```python
from build123d import *

# Parameters (mm, degrees)
EXTRUDE_2_DEPTH     = 70
CUT_EXTRUDE_1_DEPTH = 90
EXTRUDE_3_OUTLINE_R = 45
EXTRUDE_3_DEPTH     = 20
EXTRUDE_START       = -10
EXTRUDE_4_DEPTH     = 10
EXTRUDE_START_2     = -20
EXTRUDE_5_DEPTH     = 20
CUT_EXTRUDE_2_DEPTH = 207.942020866
EXTRUDE_START_3     = 35
SKETCH_13_R         = 50
EXTRUDE_6_DEPTH     = 35
CUT_EXTRUDE_START   = 15
CUT_EXTRUDE_3_DEPTH = 15
SKETCH_15_R         = 6.5
CUT_EXTRUDE_4_DEPTH = 207.942020866
CUT_EXTRUDE_5_REACH = 207.305


# Read off the part's stored shape, not the designer's step: the extrude step
with BuildPart() as part:
    # Sketch 1 → Extrude 2 (new body)
    with BuildSketch(Plane(origin=(0, 0, 0), x_dir=(1, 0, 0), z_dir=(0, 1, 0))):
        with BuildLine():
            Line((8.235294118, 69.513883008), (92.058823529, 59.583328292))
            ThreePointArc((92.058823529, 59.583328292), (145, 0), (92.058823529, -59.583328292))
            Line((92.058823529, -59.583328292), (8.235294118, -69.513883008))
            ThreePointArc((8.235294118, -69.513883008), (-70, 0), (8.235294118, 69.513883008))
        make_face()
    extrude(amount=EXTRUDE_2_DEPTH)

    # Sketch 2 → Cut-Extrude 1 (cut)
    with BuildSketch(Plane(origin=(0, 70, 0), x_dir=(1, 0, 0), z_dir=(0, 1, 0))):
        with BuildLine():
            Line((7.058823529, -59.583328292), (90.882352941, -49.652773577))
            ThreePointArc((90.882352941, -49.652773577), (135, 0), (90.882352941, 49.652773577))
            Line((90.882352941, 49.652773577), (7.058823529, 59.583328292))
            ThreePointArc((7.058823529, 59.583328292), (-60, 0), (7.058823529, -59.583328292))
        make_face()
    extrude(amount=-CUT_EXTRUDE_1_DEPTH, mode=Mode.SUBTRACT)



with BuildPart() as body_2:
    # Extrude 3 outline → Extrude 3 (new body)
    with BuildSketch(Plane.XZ):
        with BuildLine():
            ThreePointArc((90.882352941, -49.652773577), (135, 0), (90.882352941, 49.652773577))
            Line((90.882352941, 49.652773577), (68.128593603, 52.348406339))
            ThreePointArc((68.128593603, 52.348406339), (30, 0), (68.128593603, -52.348406339))
            Line((68.128593603, -52.348406339), (90.882352941, -49.652773577))
        make_face()
        with Locations((85, 0)):
            Circle(EXTRUDE_3_OUTLINE_R, mode=Mode.SUBTRACT)
    extrude(amount=EXTRUDE_3_DEPTH)


with BuildPart() as part_1:
    add(part.part)

    add(body_2.part)  # Extrude 4 merges body 2
    # Sketch 8 → Extrude 4 (add)
    with BuildSketch(Plane.XZ.offset(EXTRUDE_START)):
        with BuildLine():
            Line((90.882352941, -49.652773577), (7.058823529, -59.583328292))
            ThreePointArc((7.058823529, -59.583328292), (-60, 0), (7.058823529, 59.583328292))
            Line((7.058823529, 59.583328292), (90.882352941, 49.652773577))
            ThreePointArc((90.882352941, 49.652773577), (135, 0), (90.882352941, -49.652773577))
        make_face()
    extrude(amount=EXTRUDE_4_DEPTH)

    # Sketch 9 → Extrude 5 (add)
    with BuildSketch(Plane(origin=(0, 70, 0), x_dir=(1, 0, 0), z_dir=(0, 1, 0)).offset(EXTRUDE_START_2)):
        with BuildLine():
            Line((11.176470588, 94.340269796), (95, 84.409715081))
            ThreePointArc((95, 84.409715081), (170, 0), (95, -84.409715081))
            Line((95, -84.409715081), (11.176470588, -94.340269796))
            ThreePointArc((11.176470588, -94.340269796), (-95, 0), (11.176470588, 94.340269796))
        make_face()
        with BuildLine():
            Line((8.235294118, -69.513883008), (92.058823529, -59.583328292))
            ThreePointArc((92.058823529, -59.583328292), (145, 0), (92.058823529, 59.583328292))
            Line((92.058823529, 59.583328292), (8.235294118, 69.513883008))
            ThreePointArc((8.235294118, 69.513883008), (-70, 0), (8.235294118, -69.513883008))
        make_face(mode=Mode.SUBTRACT)
    extrude(amount=EXTRUDE_5_DEPTH)

    # Sketch 10 → Cut-Extrude 2 (cut, through all)
    with BuildSketch(Plane.XZ.offset(-50)):
        with BuildLine():
            ThreePointArc((88.858252054, 75.067395659), (93.152609723, 69.524378153), (98.766439672, 73.725742714))
            ThreePointArc((98.766439672, 73.725742714), (96.301264767, 74.143653907), (93.823529412, 74.479160365))
            Line((93.823529412, 74.479160365), (88.858252054, 75.067395659))
        make_face()
        with BuildLine():
            ThreePointArc((93.823529412, 74.479160365), (96.301264767, 74.143653907), (98.766439672, 73.725742714))
            ThreePointArc((98.766439672, 73.725742714), (98.809236548, 74.101371603), (98.823529412, 74.479160365))
            ThreePointArc((98.823529412, 74.479160365), (94.11815902, 79.470472156), (88.858252054, 75.067395659))
            Line((88.858252054, 75.067395659), (93.823529412, 74.479160365))
        make_face()
        with BuildLine():
            ThreePointArc((88.858252054, 75.067395659), (93.152609723, 69.524378153), (98.766439672, 73.725742714))
            ThreePointArc((98.766439672, 73.725742714), (96.301264767, 74.143653907), (93.823529412, 74.479160365))
            Line((93.823529412, 74.479160365), (88.858252054, 75.067395659))
        make_face()
        with BuildLine():
            ThreePointArc((93.823529412, 74.479160365), (96.301264767, 74.143653907), (98.766439672, 73.725742714))
            ThreePointArc((98.766439672, 73.725742714), (98.809236548, 74.101371603), (98.823529412, 74.479160365))
            ThreePointArc((98.823529412, 74.479160365), (94.11815902, 79.470472156), (88.858252054, 75.067395659))
            Line((88.858252054, 75.067395659), (93.823529412, 74.479160365))
        make_face()
        with BuildLine():
            ThreePointArc((10, 84.409715081), (7.513035126, 84.667315436), (5.01956968, 84.851658323))
            ThreePointArc((5.01956968, 84.851658323), (9.484855013, 79.436323316), (14.965277358, 83.821479787))
            Line((14.965277358, 83.821479787), (10, 84.409715081))
        make_face()
        with BuildLine():
            ThreePointArc((15, 84.409715081), (10.221188156, 89.404820265), (5.01956968, 84.851658323))
            ThreePointArc((5.01956968, 84.851658323), (7.513035126, 84.667315436), (10, 84.409715081))
            Line((10, 84.409715081), (14.965277358, 83.821479787))
            ThreePointArc((14.965277358, 83.821479787), (14.991311791, 84.115085473), (15, 84.409715081))
        make_face()
        with BuildLine():
            ThreePointArc((10, 84.409715081), (7.513035126, 84.667315436), (5.01956968, 84.851658323))
            ThreePointArc((5.01956968, 84.851658323), (9.484855013, 79.436323316), (14.965277358, 83.821479787))
            Line((14.965277358, 83.821479787), (10, 84.409715081))
        make_face()
        with BuildLine():
            ThreePointArc((15, 84.409715081), (10.221188156, 89.404820265), (5.01956968, 84.851658323))
            ThreePointArc((5.01956968, 84.851658323), (7.513035126, 84.667315436), (10, 84.409715081))
            Line((10, 84.409715081), (14.965277358, 83.821479787))
            ThreePointArc((14.965277358, 83.821479787), (14.991311791, 84.115085473), (15, 84.409715081))
        make_face()
        with BuildLine():
            ThreePointArc((5.01956968, -84.851658323), (7.513035126, -84.667315436), (10, -84.409715081))
            Line((10, -84.409715081), (14.965277358, -83.821479787))
            ThreePointArc((14.965277358, -83.821479787), (9.484855013, -79.436323316), (5.01956968, -84.851658323))
        make_face()
        with BuildLine():
            Line((14.965277358, -83.821479787), (10, -84.409715081))
            ThreePointArc((10, -84.409715081), (7.513035126, -84.667315436), (5.01956968, -84.851658323))
            ThreePointArc((5.01956968, -84.851658323), (10.221188156, -89.404820265), (15, -84.409715081))
            ThreePointArc((15, -84.409715081), (14.991311791, -84.115085473), (14.965277358, -83.821479787))
        make_face()
        with BuildLine():
            ThreePointArc((5.01956968, -84.851658323), (7.513035126, -84.667315436), (10, -84.409715081))
            Line((10, -84.409715081), (14.965277358, -83.821479787))
            ThreePointArc((14.965277358, -83.821479787), (9.484855013, -79.436323316), (5.01956968, -84.851658323))
        make_face()
        with BuildLine():
            Line((14.965277358, -83.821479787), (10, -84.409715081))
            ThreePointArc((10, -84.409715081), (7.513035126, -84.667315436), (5.01956968, -84.851658323))
            ThreePointArc((5.01956968, -84.851658323), (10.221188156, -89.404820265), (15, -84.409715081))
            ThreePointArc((15, -84.409715081), (14.991311791, -84.115085473), (14.965277358, -83.821479787))
        make_face()
        with BuildLine():
            ThreePointArc((98.766439672, -73.725742714), (93.152609723, -69.524378153), (88.858252054, -75.067395659))
            Line((88.858252054, -75.067395659), (93.823529412, -74.479160365))
            ThreePointArc((93.823529412, -74.479160365), (96.301264767, -74.143653907), (98.766439672, -73.725742714))
        make_face()
        with BuildLine():
            Line((93.823529412, -74.479160365), (88.858252054, -75.067395659))
            ThreePointArc((88.858252054, -75.067395659), (94.11815902, -79.470472156), (98.823529412, -74.479160365))
            ThreePointArc((98.823529412, -74.479160365), (98.809236548, -74.101371603), (98.766439672, -73.725742714))
            ThreePointArc((98.766439672, -73.725742714), (96.301264767, -74.143653907), (93.823529412, -74.479160365))
        make_face()
        with BuildLine():
            ThreePointArc((98.766439672, -73.725742714), (93.152609723, -69.524378153), (88.858252054, -75.067395659))
            Line((88.858252054, -75.067395659), (93.823529412, -74.479160365))
            ThreePointArc((93.823529412, -74.479160365), (96.301264767, -74.143653907), (98.766439672, -73.725742714))
        make_face()
        with BuildLine():
            Line((93.823529412, -74.479160365), (88.858252054, -75.067395659))
            ThreePointArc((88.858252054, -75.067395659), (94.11815902, -79.470472156), (98.823529412, -74.479160365))
            ThreePointArc((98.823529412, -74.479160365), (98.809236548, -74.101371603), (98.766439672, -73.725742714))
            ThreePointArc((98.766439672, -73.725742714), (96.301264767, -74.143653907), (93.823529412, -74.479160365))
        make_face()
    extrude(amount=-CUT_EXTRUDE_2_DEPTH, mode=Mode.SUBTRACT)

    # Sketch 13 → Extrude 6 (add)
    with BuildSketch(Plane(origin=(0, 10, 0), x_dir=(1, 0, 0), z_dir=(0, 1, 0)).offset(EXTRUDE_START_3)):
        with Locations((85, 0)):
            Circle(SKETCH_13_R)
    extrude(amount=-EXTRUDE_6_DEPTH)

    # Sketch 14 → Cut-Extrude 3 (cut)
    with BuildSketch(Plane(origin=(0, 10, 0), x_dir=(1, 0, 0), z_dir=(0, 1, 0)).offset(CUT_EXTRUDE_START)):
        with BuildLine():
            ThreePointArc((90.882352941, -49.652773577), (135, 0), (90.882352941, 49.652773577))
            ThreePointArc((90.882352941, 49.652773577), (35, 0), (90.882352941, -49.652773577))
        make_face()
    extrude(amount=-CUT_EXTRUDE_3_DEPTH, mode=Mode.SUBTRACT)

    # Sketch 15 → Cut-Extrude 4 (cut, through all)
    with BuildSketch(Plane.XZ):
        with Locations(Location((85, 0, 0), (0, 0, 90))):
            Circle(SKETCH_15_R)
    extrude(amount=-CUT_EXTRUDE_4_DEPTH, mode=Mode.SUBTRACT)

    # Sketch 16 → Cut-Extrude 5 (cut, up to next)
    with BuildSketch(Plane(origin=(0, 45, 0), x_dir=(1, 0, 0), z_dir=(0, 1, 0)), mode=Mode.PRIVATE) as cut_extrude_5_sk1:
        with BuildLine():
            Line((60, 0), (60, 43.301270189))
            ThreePointArc((60, 43.301270189), (41.698729811, 25), (35, 0))
            Line((35, 0), (60, 0))
        make_face()
    cut_extrude_5_tool1 = extrude(cut_extrude_5_sk1.sketch, amount=-CUT_EXTRUDE_5_REACH, mode=Mode.PRIVATE) & part_1.part
    # Sketch 16 → Cut-Extrude 5 (cut, up to next)
    with BuildSketch(Plane(origin=(0, 45, 0), x_dir=(1, 0, 0), z_dir=(0, 1, 0)), mode=Mode.PRIVATE) as cut_extrude_5_sk2:
        with BuildLine():
            ThreePointArc((35, 0), (41.698729811, -25), (60, -43.301270189))
            Line((60, -43.301270189), (60, 0))
            Line((60, 0), (35, 0))
        make_face()
    cut_extrude_5_tool2 = extrude(cut_extrude_5_sk2.sketch, amount=-CUT_EXTRUDE_5_REACH, mode=Mode.PRIVATE) & part_1.part
    # Sketch 16 → Cut-Extrude 5 (cut, up to next)
    with BuildSketch(Plane(origin=(0, 45, 0), x_dir=(1, 0, 0), z_dir=(0, 1, 0)), mode=Mode.PRIVATE) as cut_extrude_5_sk3:
        with BuildLine():
            Line((60, 0), (60, 43.301270189))
            ThreePointArc((60, 43.301270189), (41.698729811, 25), (35, 0))
            Line((35, 0), (60, 0))
        make_face()
    cut_extrude_5_tool3 = extrude(cut_extrude_5_sk3.sketch, amount=-CUT_EXTRUDE_5_REACH, mode=Mode.PRIVATE) & part_1.part
    # Sketch 16 → Cut-Extrude 5 (cut, up to next)
    with BuildSketch(Plane(origin=(0, 45, 0), x_dir=(1, 0, 0), z_dir=(0, 1, 0)), mode=Mode.PRIVATE) as cut_extrude_5_sk4:
        with BuildLine():
            ThreePointArc((35, 0), (41.698729811, -25), (60, -43.301270189))
            Line((60, -43.301270189), (60, 0))
            Line((60, 0), (35, 0))
        make_face()
    cut_extrude_5_tool4 = extrude(cut_extrude_5_sk4.sketch, amount=-CUT_EXTRUDE_5_REACH, mode=Mode.PRIVATE) & part_1.part
    add(cut_extrude_5_tool1.solids().sort_by_distance((49.748992, 45, -16.960149))[0], mode=Mode.SUBTRACT)
    add(cut_extrude_5_tool2.solids().sort_by_distance((49.748992, 45, 16.960149))[0], mode=Mode.SUBTRACT)
    add(cut_extrude_5_tool3.solids().sort_by_distance((49.748992, 45, -16.960149))[0], mode=Mode.SUBTRACT)
    add(cut_extrude_5_tool4.solids().sort_by_distance((49.748992, 45, 16.960149))[0], mode=Mode.SUBTRACT)


solid = part_1.part
```
CAD build for the part. Positions are in the model's coordinates, mm. A direction names the side the tool comes from. Round coordinates to 2 decimals unless told otherwise and drop trailing zeros. Order: outer loops, then holes, each group sorted by start corner. A loop starts at its lowest first (then second) coordinate and runs counter-clockwise, first axis right, second up. Notation, with made-up numbers: (-14, -36) - (-4, -36) arc R18 cw to (-4, -13) - close; hole circle Ø2 at (-12, 50.25). An arc over 180 degrees is marked (long way). Answer as CSV lines item,"result". Start each with the question number.
1. Pin check, flat tips, straight feed: pin 1 (1.5 mm diameter, centred on x = -57, z = -1, fed in from +Y); pin 2 (4 mm diameter, centred on x = -23.5, z = 5, fed in from -Y); pin 3 (2 mm diameter, centred on x = 131.5, z = 57, fed in from -Y); pin 4 (11.5 mm diameter, centred on x = 85, z = 0, fed in from +Y). Stop position of each tip, or through.
2. Tool access for faces 4 (the face through (15, 0, -1)), 5 (the face through (97, 45, -1)), 6 (the face through (97, 25, -1)): list every direction of +Z, -Z, +X, -X, +Y, -Y with a clear straight run to the whole face (end or side of a thin tool).
3. Pull direction Y, two halves, no side cores. Call faces 1 (the face through (91.345, 4.93, -1.409)), 2 (the face through (39, -20, 0)), 3 (the face through (39, 10, 1)): +Y half, -Y half, draft (parallel to the pull), parting line (faces both ways), or undercut.
4. Saw through at C-C, the plane y = -3.5. Write the cut outline in (x, z).
5. Saw through at B-B, the plane x = 85. Count the separate pieces of the cut face and the enclosed holes in it, and give its area (3 significant figures).
6. Saw through at A-A, the plane x = 0. Write the cut outline in (y, z), and give its area (3 significant figures).
7. Drill centre lines: L1, parallel to Z at x = 0, y = 43.5; L2, parallel to Z at x = 64, y = 37; L3, parallel to X at y = 31, z = 0. Where is each one in solid material? Low to high. Write a range as [from, to].
8. Saw through at D-D, the plane z = -37. Write the cut outline in (x, y), and give its area (3 significant figures).
Model answer:
1,pin 1,"stops at y = 10"
1,pin 2,"stops at y = 0"
1,pin 3,"stops at y = 50"
1,pin 4,"passes through"
2,face 4,"-Y"
2,face 5,"+Y"
2,face 6,"none"
3,face 1,"draft"
3,face 2,"-Y half"
3,face 3,"undercut"
4,outline,"(68.13, -52.35) - (90.88, -49.65) arc R50 ccw to (90.88, 49.65) - (68.13, 52.35) arc R55 ccw to start; hole circle Ø90 at (85, 0)"
5,separate pieces,"4"
5,enclosed holes,"0"
5,area,"5,250 mm²"
6,outline,"(0, -70) - (50, -70) - (50, -95) - (70, -95) - (70, -60) - (10, -60) - (10, 60) - (70, 60) - (70, 95) - (50, 95) - (50, 70) - (0, 70) - close"
6,area,"3,600 mm²"
7,L1,"z = [-70, -60], [60, 70]"
7,L2,"z = [-62.91, -52.84], [-45.38, 45.38], [52.84, 62.91]"
7,L3,"x = [-70, -60], [60, 78.5], [91.5, 145]"
8,outline,"(-87.5, 50) - (-59.42, 50) - (-59.42, 0) - (44.31, 0) - (44.31, -20) - (59.39, -20) - (59.39, 0) - (110.61, 0) - (110.61, -20) - (118.63, -20) - (118.63, 0) - (132.23, 0) - (132.23, 50) - (161.52, 50) - (161.52, 70) - (118.63, 70) - (118.63, 45) - (60, 45) - (60, 25) - (118.63, 25) - (118.63, 10) - (-47.23, 10) - (-47.23, 70) - (-87.5, 70) - close"
8,area,"6,250 mm²"
